For this review, take the finished solid that the model builds, in its own axes (mm). A direction names the side the tool comes from. Coordinates: 2 decimals unless noted, no trailing zeros. Loops run counter-clockwise (first coordinate to the right, second up) from the corner with the lowest first, then second, coordinate; pieces in that order, holes last. Notation, with made-up numbers: (68, -19) -> (122, -19) arc R31 ccw to (122, 13) -> close; hole circle Ø6 at (15, -29). An arc over 180 degrees is marked (long way). One line per item, written item: value.
from build123d import *

# Parameters (mm, degrees)
F0_R     = 2.5
F0_R_2   = 3.05
F1_DEPTH = 8
F2_DEPTH = 2


with BuildPart() as f1:
    # F0 (on Top) → F1 (new body)
    with BuildSketch(Plane.XY):
        with BuildLine():
            Line((30.5, 0), (160, 0))
            ThreePointArc((160, 0), (113.137085, 113.137085), (0, 160))
            Line((0, 160), (0, 30.5))
            ThreePointArc((0, 30.5), (21.566757, 21.566757), (30.5, 0))
        make_face()
        with Locations((32.335784, 13.39392)):
            Circle(F0_R, mode=Mode.SUBTRACT)
        with Locations((13.39392, 32.335784)):
            Circle(F0_R, mode=Mode.SUBTRACT)
        with Locations((27.718586, 27.718586)):
            Circle(F0_R_2, mode=Mode.SUBTRACT)
        with Locations((50.813374, 21.047589)):
            Circle(F0_R, mode=Mode.SUBTRACT)
        with Locations((69.290965, 28.701257)):
            Circle(F0_R, mode=Mode.SUBTRACT)
        with Locations((21.047589, 50.813374)):
            Circle(F0_R, mode=Mode.SUBTRACT)
        with Locations((28.701257, 69.290965)):
            Circle(F0_R, mode=Mode.SUBTRACT)
        with Locations((87.768556, 36.354926)):
            Circle(F0_R, mode=Mode.SUBTRACT)
        with Locations((106.246146, 44.008595)):
            Circle(F0_R, mode=Mode.SUBTRACT)
        with Locations((124.723737, 51.662263)):
            Circle(F0_R, mode=Mode.SUBTRACT)
        with Locations((143.201328, 59.315932)):
            Circle(F0_R, mode=Mode.SUBTRACT)
        with Locations((36.354926, 87.768556)):
            Circle(F0_R, mode=Mode.SUBTRACT)
        with Locations((44.008595, 106.246146)):
            Circle(F0_R, mode=Mode.SUBTRACT)
        with Locations((51.662263, 124.723737)):
            Circle(F0_R, mode=Mode.SUBTRACT)
        with Locations((59.315932, 143.201328)):
            Circle(F0_R, mode=Mode.SUBTRACT)
        with BuildLine():
            Line((3, 0), (26.5, 0))
            ThreePointArc((26.5, 0), (18.73833, 18.73833), (0, 26.5))
            Line((0, 26.5), (0, 3))
            ThreePointArc((0, 3), (2.12132, 2.12132), (3, 0))
        make_face()
        with Locations((10.253048, 10.253048)):
            Circle(F0_R_2, mode=Mode.SUBTRACT)
        with BuildLine():
            Line((26.5, 0), (30.5, 0))
            ThreePointArc((30.5, 0), (21.566757, 21.566757), (0, 30.5))
            Line((0, 30.5), (0, 26.5))
            ThreePointArc((0, 26.5), (18.73833, 18.73833), (26.5, 0))
        make_face()
    extrude(amount=-F1_DEPTH)

    # F0 (on Top) → F2 (cut)
    with BuildSketch(Plane.XY):
        with BuildLine():
            Line((26.5, 0), (30.5, 0))
            ThreePointArc((30.5, 0), (21.566757, 21.566757), (0, 30.5))
            Line((0, 30.5), (0, 26.5))
            ThreePointArc((0, 26.5), (18.73833, 18.73833), (26.5, 0))
        make_face()
    extrude(amount=-F2_DEPTH, mode=Mode.SUBTRACT)


solid = f1.part
1. To check wall thickness, follow probe 1 along X at (y, z) = (11.5, -7.25); probe 2 along X at (y, z) = (34.5, -2); probe 3 along X at (y, z) = (68, -1.75). State the ranges of each line that lie inside material, in increasing order. Write a range as from..to.
Return value:
probe 1: x = 0..7.47, 13.04..30.7, 33.97..159.59
probe 2: x = 0..12.14, 14.65..86.09, 89.44..156.24
probe 3: x = 0..26.56, 30.84..144.83
2. Insertion check: pin 1 Ø1 at (y, z) = (61, -2) entering from +X. The pin has a flat end and moves straight along its axis. Give the tip position at first contact, or say it passes through.
Return value:
pin 1: stops at x = 148.12
3. Take a section at B-B, the plane z = -6.75. Give the number of separate pieces and of enclosed holes in the cut face, and give its area (3 significant figures).
Return value:
separate pieces: 1
enclosed holes: 16
area: 19,800 mm2
4. For faces 5 (the cylindrical face through (18.531, 18.943, -0.986)), 6 (the flat face through (80, 0, -4)), list the 3-axis set-ups (+Z, -Z, +X, -X, +Y, -Y) from which the entire face can be reached by the end or side of a thin tool; tool diameter is ignored.
Return value:
face 5: +Z
face 6: +Z, -Z, +X, -X, -Y
5. Take a section at C-C, the plane x = 111.5. Give the boundary of the cut face in (y, z), and give its area (3 significant figures).
Return value:
outline: (0, -8) -> (114.75, -8) -> (114.75, 0) -> (0, 0) -> close
area: 918 mm2
6. Take a section at A-A, the plane x = 143. Give the boundary of the cut face in (y, z).
Return value:
outline: (0, -8) -> (56.82, -8) -> (56.82, 0) -> (0, 0) -> close; (61.81, -8) -> (71.77, -8) -> (71.77, 0) -> (61.81, 0) -> close
7. The part is to be moulded in two halves that separate along Y. For faces 1 (the cylindrical face through (114.37, 111.89, -3.94)), 2 (the cylindrical face through (41.51, 106.36, -3.94)), 3 (the cylindrical face through (70.44, 26.48, -3.94)), 4 (the flat face through (79, 81, 0)), say which applies: pulls with the +Y half, pulls with the -Y half, needs draft (parallel to the pull), parting line crosses it, or undercut.
Return value:
face 1: pulls with the +Y half
face 2: undercut
face 3: undercut
face 4: needs draft
